from build123d import *

# Parameters (mm, degrees)
SKETCH1_W           = 350
SKETCH1_H           = 300
BOSS_EXTRUDE1_DEPTH = 3
SKETCH1_3_R         = 4
BOSS_EXTRUDE2_DEPTH = 15
BOSS_EXTRUDE3_START = -150
BOSS_EXTRUDE3_DEPTH = 150
CUT_EXTRUDE1_DEPTH  = 150


# Read off the part's stored shape, not the designer's step: Boss-Extrude3
with BuildPart() as part:
    # Sketch1 → Boss-Extrude1 (new body)
    with BuildSketch(Plane(origin=(0, 0, 0), x_dir=(1, 0, 0), z_dir=(0, 1, 0))):
        Rectangle(SKETCH1_W, SKETCH1_H)
    extrude(amount=-BOSS_EXTRUDE1_DEPTH)

    # Sketch1_3 → Boss-Extrude2 (add)
    with BuildSketch(Plane(origin=(0, 0, 0), x_dir=(1, 0, 0), z_dir=(0, 1, 0))):
        with Locations(Location((0, 52.5, 0), (0, 0, 270))):
            Circle(SKETCH1_3_R)
        with Locations(Location((52.5, 0, 0), (0, 0, 270))):
            Circle(SKETCH1_3_R)
        with Locations(Location((0, -52.5, 0), (0, 0, 270))):
            Circle(SKETCH1_3_R)
        with Locations(Location((-52.5, 0, 0), (0, 0, 270))):
            Circle(SKETCH1_3_R)
    extrude(amount=BOSS_EXTRUDE2_DEPTH)

    # Boss-Extrude3 outline → Boss-Extrude3 (add)
    with BuildSketch(Plane(origin=(0, 0, 0), x_dir=(1, 0, 0), z_dir=(0, 1, 0)).offset(BOSS_EXTRUDE3_START)):
        with BuildLine():
            Line((-192.5, 127.5), (-175, 127.5))
            Line((-175, 127.5), (-175, -127.5))
            Line((-175, -127.5), (-192.5, -127.5))
            ThreePointArc((-192.5, -127.5), (-196.035533906, -128.964466094), (-197.5, -132.5))
            Line((-197.5, -132.5), (-197.5, -167.5))
            ThreePointArc((-197.5, -167.5), (-196.035533906, -171.035533906), (-192.5, -172.5))
            Line((-192.5, -172.5), (-157.5, -172.5))
            ThreePointArc((-157.5, -172.5), (-153.964466094, -171.035533906), (-152.5, -167.5))
            Line((-152.5, -167.5), (-152.5, -150))
            Line((-152.5, -150), (152.5, -150))
            Line((152.5, -150), (152.5, -167.5))
            ThreePointArc((152.5, -167.5), (153.964466094, -171.035533906), (157.5, -172.5))
            Line((157.5, -172.5), (192.5, -172.5))
            ThreePointArc((192.5, -172.5), (196.035533906, -171.035533906), (197.5, -167.5))
            Line((197.5, -167.5), (197.5, -132.5))
            ThreePointArc((197.5, -132.5), (196.035533906, -128.964466094), (192.5, -127.5))
            Line((192.5, -127.5), (175, -127.5))
            Line((175, -127.5), (175, 127.5))
            Line((175, 127.5), (192.5, 127.5))
            ThreePointArc((192.5, 127.5), (196.035533906, 128.964466094), (197.5, 132.5))
            Line((197.5, 132.5), (197.5, 167.5))
            ThreePointArc((197.5, 167.5), (196.035533906, 171.035533906), (192.5, 172.5))
            Line((192.5, 172.5), (157.5, 172.5))
            ThreePointArc((157.5, 172.5), (153.964466094, 171.035533906), (152.5, 167.5))
            Line((152.5, 167.5), (152.5, 150))
            Line((152.5, 150), (-152.5, 150))
            Line((-152.5, 150), (-152.5, 167.5))
            ThreePointArc((-152.5, 167.5), (-153.964466094, 171.035533906), (-157.5, 172.5))
            Line((-157.5, 172.5), (-192.5, 172.5))
            ThreePointArc((-192.5, 172.5), (-196.035533906, 171.035533906), (-197.5, 167.5))
            Line((-197.5, 167.5), (-197.5, 132.5))
            ThreePointArc((-197.5, 132.5), (-196.035533906, 128.964466094), (-192.5, 127.5))
        make_face()
        with BuildLine():
            ThreePointArc((157.5, -127.5), (153.964466094, -128.964466094), (152.5, -132.5))
            Line((152.5, -132.5), (152.5, -145))
            Line((152.5, -145), (-152.5, -145))
            Line((-152.5, -145), (-152.5, -132.5))
            ThreePointArc((-152.5, -132.5), (-153.964466094, -128.964466094), (-157.5, -127.5))
            Line((-157.5, -127.5), (-170, -127.5))
            Line((-170, -127.5), (-170, 127.5))
            Line((-170, 127.5), (-157.5, 127.5))
            ThreePointArc((-157.5, 127.5), (-153.964466094, 128.964466094), (-152.5, 132.5))
            Line((-152.5, 132.5), (-152.5, 145))
            Line((-152.5, 145), (152.5, 145))
            Line((152.5, 145), (152.5, 132.5))
            ThreePointArc((152.5, 132.5), (153.964466094, 128.964466094), (157.5, 127.5))
            Line((157.5, 127.5), (170, 127.5))
            Line((170, 127.5), (170, -127.5))
            Line((170, -127.5), (157.5, -127.5))
        make_face(mode=Mode.SUBTRACT)
    extrude(amount=BOSS_EXTRUDE3_DEPTH)

    # Sketch3 → Cut-Extrude1 (cut)
    with BuildSketch(Plane.ZY.offset(175)):
        with BuildLine():
            Line((-83.359623482, -64.977900186), (-87.265323275, -62.72294336))
            ThreePointArc((-87.265323275, -62.72294336), (-90.673265007, -77.210943421), (-87.265323275, -91.698943483))
            Line((-87.265323275, -91.698943483), (-83.359623482, -89.443986656))
            ThreePointArc((-83.359623482, -89.443986656), (-86.173265007, -77.210943421), (-83.359623482, -64.977900186))
        make_face()
        with BuildLine():
            Line((-72.047295017, -71.50907607), (-80.754099181, -66.482200343))
            ThreePointArc((-80.754099181, -66.482200343), (-83.173265007, -77.210943421), (-80.754099181, -87.939686499))
            Line((-80.754099181, -87.939686499), (-72.047295017, -82.912810772))
            ThreePointArc((-72.047295017, -82.912810772), (-73.173265007, -77.210943421), (-72.047295017, -71.50907607))
        make_face()
        with BuildLine():
            ThreePointArc((-60.172318038, -52.290995849), (-70.673265007, -55.560308327), (-78.75504615, -63.019738928))
            Line((-78.75504615, -63.019738928), (-70.048241987, -68.046614655))
            ThreePointArc((-70.048241987, -68.046614655), (-65.673265007, -64.220562364), (-60.172318038, -62.344747304))
            Line((-60.172318038, -62.344747304), (-60.172318038, -52.290995849))
        make_face()
        with BuildLine():
            ThreePointArc((-60.172318038, -44.772481883), (-74.423265007, -49.065117798), (-85.266270244, -59.260481944))
            Line((-85.266270244, -59.260481944), (-81.360570452, -61.515438771))
            ThreePointArc((-81.360570452, -61.515438771), (-72.173265007, -52.962232115), (-60.172318038, -49.282395536))
            Line((-60.172318038, -49.282395536), (-60.172318038, -44.772481883))
        make_face()
        with BuildLine():
            ThreePointArc((-31.080259771, -59.260481944), (-41.923265007, -49.065117798), (-56.174211977, -44.772481883))
            Line((-56.174211977, -44.772481883), (-56.174211977, -49.282395536))
            ThreePointArc((-56.174211977, -49.282395536), (-44.173265007, -52.962232115), (-34.985959563, -61.515438771))
            Line((-34.985959563, -61.515438771), (-31.080259771, -59.260481944))
        make_face()
        with BuildLine():
            ThreePointArc((-37.591483864, -63.019738928), (-45.673265007, -55.560308327), (-56.174211977, -52.290995849))
            Line((-56.174211977, -52.290995849), (-56.174211977, -62.344747304))
            ThreePointArc((-56.174211977, -62.344747304), (-50.673265007, -64.220562364), (-46.298288028, -68.046614655))
            Line((-46.298288028, -68.046614655), (-37.591483864, -63.019738928))
        make_face()
        with BuildLine():
            ThreePointArc((-48.925702168, -69.563552916), (-52.173265007, -66.818638576), (-56.174211977, -65.378623827))
            Line((-56.174211977, -65.378623827), (-56.174211977, -72.627954551))
            ThreePointArc((-56.174211977, -72.627954551), (-55.673265007, -72.880816402), (-55.203806736, -73.188218278))
            Line((-55.203806736, -73.188218278), (-48.925702168, -69.563552916))
        make_face()
        with BuildLine():
            ThreePointArc((-60.172318038, -65.378623827), (-64.173265007, -66.818638576), (-67.420827847, -69.563552916))
            Line((-67.420827847, -69.563552916), (-61.142723279, -73.188218278))
            ThreePointArc((-61.142723279, -73.188218278), (-60.673265007, -72.880816402), (-60.172318038, -72.627954551))
            Line((-60.172318038, -72.627954551), (-60.172318038, -65.378623827))
        make_face()
        with BuildLine():
            Line((-63.141776309, -76.650679694), (-69.419880877, -73.026014332))
            ThreePointArc((-69.419880877, -73.026014332), (-70.173265007, -77.210943421), (-69.419880877, -81.395872511))
            Line((-69.419880877, -81.395872511), (-63.141776309, -77.771207148))
            ThreePointArc((-63.141776309, -77.771207148), (-63.173265007, -77.210943421), (-63.141776309, -76.650679694))
        make_face()
        with BuildLine():
            Line((-61.142723279, -81.233668564), (-67.420827847, -84.858333926))
            ThreePointArc((-67.420827847, -84.858333926), (-64.173265007, -87.603248267), (-60.172318038, -89.043263015))
            Line((-60.172318038, -89.043263015), (-60.172318038, -81.793932291))
            ThreePointArc((-60.172318038, -81.793932291), (-60.673265007, -81.54107044), (-61.142723279, -81.233668564))
        make_face()
        with BuildLine():
            Line((-56.174211977, -81.793932291), (-56.174211977, -89.043263015))
            ThreePointArc((-56.174211977, -89.043263015), (-52.173265007, -87.603248267), (-48.925702168, -84.858333926))
            Line((-48.925702168, -84.858333926), (-55.203806736, -81.233668564))
            ThreePointArc((-55.203806736, -81.233668564), (-55.673265007, -81.54107044), (-56.174211977, -81.793932291))
        make_face()
        with BuildLine():
            ThreePointArc((-46.926649138, -81.395872511), (-46.173265007, -77.210943421), (-46.926649138, -73.026014332))
            Line((-46.926649138, -73.026014332), (-53.204753706, -76.650679694))
            ThreePointArc((-53.204753706, -76.650679694), (-53.181143389, -76.930369464), (-53.173265007, -77.210943421))
            ThreePointArc((-53.173265007, -77.210943421), (-53.181143389, -77.491517379), (-53.204753706, -77.771207148))
            Line((-53.204753706, -77.771207148), (-46.926649138, -81.395872511))
        make_face()
        with BuildLine():
            ThreePointArc((-35.592430834, -87.939686499), (-33.173265007, -77.210943421), (-35.592430834, -66.482200343))
            Line((-35.592430834, -66.482200343), (-44.299234997, -71.50907607))
            ThreePointArc((-44.299234997, -71.50907607), (-43.173265007, -77.210943421), (-44.299234997, -82.912810772))
            Line((-44.299234997, -82.912810772), (-35.592430834, -87.939686499))
        make_face()
        with BuildLine():
            ThreePointArc((-25.673265007, -77.210943421), (-26.536720524, -69.769233056), (-29.08120674, -62.72294336))
            Line((-29.08120674, -62.72294336), (-32.986906533, -64.977900186))
            ThreePointArc((-32.986906533, -64.977900186), (-30.173265007, -77.210943421), (-32.986906533, -89.443986656))
            Line((-32.986906533, -89.443986656), (-29.08120674, -91.698943483))
            ThreePointArc((-29.08120674, -91.698943483), (-26.536720524, -84.652653786), (-25.673265007, -77.210943421))
        make_face()
        with BuildLine():
            Line((-56.174211977, -105.139491306), (-56.174211977, -109.64940496))
            ThreePointArc((-56.174211977, -109.64940496), (-41.923265007, -105.356769044), (-31.080259771, -95.161404898))
            Line((-31.080259771, -95.161404898), (-34.985959563, -92.906448072))
            ThreePointArc((-34.985959563, -92.906448072), (-44.173265007, -101.459654727), (-56.174211977, -105.139491306))
        make_face()
        with BuildLine():
            Line((-56.174211977, -92.077139538), (-56.174211977, -102.130890993))
            ThreePointArc((-56.174211977, -102.130890993), (-45.673265007, -98.861578516), (-37.591483864, -91.402147915))
            Line((-37.591483864, -91.402147915), (-46.298288028, -86.375272187))
            ThreePointArc((-46.298288028, -86.375272187), (-50.673265007, -90.201324478), (-56.174211977, -92.077139538))
        make_face()
        with BuildLine():
            Line((-70.048241987, -86.375272187), (-78.75504615, -91.402147915))
            ThreePointArc((-78.75504615, -91.402147915), (-70.673265007, -98.861578516), (-60.172318038, -102.130890993))
            Line((-60.172318038, -102.130890993), (-60.172318038, -92.077139538))
            ThreePointArc((-60.172318038, -92.077139538), (-65.673265007, -90.201324478), (-70.048241987, -86.375272187))
        make_face()
        with BuildLine():
            Line((-81.360570452, -92.906448072), (-85.266270244, -95.161404898))
            ThreePointArc((-85.266270244, -95.161404898), (-74.423265007, -105.356769044), (-60.172318038, -109.64940496))
            Line((-60.172318038, -109.64940496), (-60.172318038, -105.139491306))
            ThreePointArc((-60.172318038, -105.139491306), (-72.173265007, -101.459654727), (-81.360570452, -92.906448072))
        make_face()
    extrude(amount=-CUT_EXTRUDE1_DEPTH, mode=Mode.SUBTRACT)


solid = part.part
Could you check a few things on this model? Use its own coordinates, in mm. A direction names the side the tool comes from. Give positions to 0.01 mm unless a question says otherwise; leave off trailing zeros. Order: outer loops, then holes, each group sorted by start corner. A loop starts at its lowest first (then second) coordinate and runs counter-clockwise, first axis right, second up. Notation, with made-up numbers: M 29.5,-2 L 56.5,-2 A25 cw 56.5,17 Z; hole C 19,84 d10. An arc over 180 degrees is marked long. One line per question, with ' | ' between items.
1. I want a section at B-B (x = -40.5). List the corners of the cut face in (y, z) for me.
Results:
outline: M -150,-150 L 0,-150 L 0,150 L -150,150 L -150,145 L -3,145 L -3,-145 L -150,-145 Z
2. If I drill on line 1 (Z direction, x = 144.5, y = -20); line 2 (X direction, y = -107, z = 152.5); line 3 (X direction, y = -17.5, z = -102), over which ranges is the centre line in solid material (lowest first)?
Results:
line 1: -150 to -145, 145 to 150 | line 2: -197.5 to -152.5, 152.5 to 197.5 | line 3: -175 to -170, 170 to 175
3. We'd pull the mould along X, two halves only. Please class faces 4 (the face through (164, -78, 127.5)), 5 (the face through (197.5, -76, -150)), 6 (the face through (-197.5, -76, 150)): +X half, -X half, draft (parallel to the pull), parting line (faces both ways), or undercut.
Results:
face 4: undercut | face 5: +X half | face 6: -X half
4. I want a section at A-A (z = 19). List the corners of the cut face in (x, y) for me.
Results:
outline: M -175,-150 L -170,-150 L -170,-3 L 170,-3 L 170,-150 L 175,-150 L 175,0 L -175,0 Z
5. For faces 1 (the face through (-175, -76, -2)), 2 (the face through (184, -76, -127.5)), 3 (the face through (152.5, -76, 159)), which set-ups out of +Z, -Z, +X, -X, +Y, -Y let a thin tool reach every point of the face, with its end or its side?
Results:
face 1: -X, +Y, -Y | face 2: +X, +Y, -Y | face 3: +Z, +Y, -Y
6. I'm going to push flat-ended pins straight in: pin 1 (6 mm diameter, centred on y = -74, z = 99.5, fed in from +X); pin 2 (2 mm diameter, centred on x = 62.5, y = -65, fed in from +Z); pin 3 (5 mm diameter, centred on x = 144.5, z = -61.5, fed in from +Y). Where does each tip first touch, or does it pass through?
Results:
pin 1: x = 175 | pin 2: z = 150 | pin 3: y = 0
